```python
from build123d import *

# Parameters (mm, degrees)
BOSS_EXTRUDE1_DEPTH = 150


with BuildPart() as part:
    # Sketch2 → Boss-Extrude1 (new body)
    with BuildSketch(Plane(origin=(0, 0, 0), x_dir=(1, 0, 0), z_dir=(0, 1, 0))):
        Polygon((315, -100), (315, -10), (305, -10), (305, -110), (695, -110), (695, -10), (685, -10), (685, -100), align=None)
        Polygon((305, 0), (0, 0), (0, 990), (0, 1010), (0, 2000), (305, 2000), (315, 2000), (315, 2010), (305, 2010), (-10, 2010), (-10, -10), (305, -10), (315, -10), (315, 0), align=None)
        Polygon((1000, 1010), (1000, 990), (1000, 0), (695, 0), (685, 0), (685, -10), (695, -10), (1010, -10), (1010, 2010), (695, 2010), (685, 2010), (685, 2000), (695, 2000), (1000, 2000), align=None)
        Polygon((305, 2010), (315, 2010), (315, 2100), (685, 2100), (685, 2010), (695, 2010), (695, 2110), (305, 2110), align=None)
    extrude(amount=BOSS_EXTRUDE1_DEPTH)


solid = part.part
```
Geometry check sheet. Reference: the model listing, model coordinates, mm. A direction names the side the tool comes from. Coordinates: 2 decimals unless noted, no trailing zeros. Write each loop counter-clockwise with the first axis right and the second up, starting at its lowest first coordinate (ties: lowest second). Pieces come first, ordered by that corner, then holes. Notation, with made-up numbers: M 40.25,52.5 L 92.25,52.5 A24 ccw 92.25,79.5 Z; hole C 70.5,72.25 d6. An arc over 180 degrees is marked long. Use one line per item in the form item = value. Start each with the question number.
1) Set-up check for faces 5 (the flat face through (305, 74, 59)), 6 (the flat face through (695, 74, 61)), 7 (the flat face through (497, 74, -2100)): record each of +Z, -Z, +X, -X, +Y, -Y from which the full face is reachable in a straight line by a thin tool's end or side.
2) Section check A-A on x = 453.5. Enter the section's corners in (y, z).
3) Section check C-C on y = 56. Enter the section's corners in (x, z).
4) Release check for a two-part mould opening along Z. For faces 1 (the flat face through (503, 74, -2110)), 2 (the flat face through (695, 74, -2059)), 3 (the flat face through (845, 74, 0)), 4 (the flat face through (685, 74, -2051)) record: pulls with the +Z half, pulls with the -Z half, needs draft (parallel to the pull), parting line crosses it, or undercut.
5) Section check B-B on z = -1509.5. Enter the section's corners in (x, y).
6) Thickness scan on probe 1 along Z at (x, y) = (692.5, 23.5); probe 2 along X at (y, z) = (11, -1221); probe 3 along Z at (x, y) = (840, 80). Record the ranges inside material, lowest first. Write a range as from..to.
Responses:
q1.face_5 = +Z, -X, +Y, -Y
q1.face_6 = +Z, +X, +Y, -Y
q1.face_7 = +Y, -Y
q2.outline = M 0,-2110 L 150,-2110 L 150,-2100 L 0,-2100 Z; M 0,100 L 150,100 L 150,110 L 0,110 Z
q3.outline = M -10,-2010 L 305,-2010 L 305,-2110 L 695,-2110 L 695,-2010 L 1010,-2010 L 1010,10 L 695,10 L 695,110 L 305,110 L 305,10 L -10,10 Z; hole M 0,-2000 L 315,-2000 L 315,-2100 L 685,-2100 L 685,-2000 L 1000,-2000 L 1000,0 L 685,0 L 685,100 L 315,100 L 315,0 L 0,0 Z
q4.face_1 = pulls with the -Z half
q4.face_2 = needs draft
q4.face_3 = undercut
q4.face_4 = undercut
q5.outline = M -10,0 L 0,0 L 0,150 L -10,150 Z; M 1000,0 L 1010,0 L 1010,150 L 1000,150 Z
q6.probe_1 = -2110..-2000, 0..110
q6.probe_2 = -10..0, 1000..1010
q6.probe_3 = -2010..-2000, 0..10
